from build123d import *

# Parameters (mm, degrees)
BOSS_EXTRUDE1_DEPTH       = 58
SKETCH3_R                 = 2.5
SKETCH3_R_2               = 20
CUT_EXTRUDE1_DEPTH        = 58
SKETCH5_R                 = 3
CUT_EXTRUDE3_DEPTH        = 58
F_4_40_TAPPED_HOLE2_D     = 2.2606
F_4_40_TAPPED_HOLE2_DEPTH = 7.6
F_4_40_TAPPED_HOLE2_TIP   = 0.679152758
SKETCH15_R                = 3
CUT_EXTRUDE4_DEPTH        = 10
FILLET1_R                 = 2
FILLET2_R                 = 2
FILLET3_R                 = 2
FILLET4_R                 = 2


with BuildPart() as part:
    # Sketch2 → Boss-Extrude1 (new body)
    with BuildSketch(Plane.XY):
        Polygon((2, 51.896715462), (36, 51.896715462), (36, -52.603284538), (75.75, -52.603284538), (75.75, -109.603284538), (72.75, -109.603284538), (72.75, -55.603284538), (33, -55.603284538), (33, 48.896715462), (2, 48.896715462), (-29, 48.896715462), (-29, -55.603284538), (-58, -55.603284538), (-58, -109.603284538), (-61, -109.603284538), (-61, -52.603284538), (-32, -52.603284538), (-32, 51.896715462), align=None)
    extrude(amount=BOSS_EXTRUDE1_DEPTH)

    # Sketch3 → Cut-Extrude1 (cut)
    with BuildSketch(Plane(origin=(0, 51.896715462, 0), x_dir=(1, 0, 0), z_dir=(0, 1, 0))):
        with Locations((-21.5, -5.5)):
            Circle(SKETCH3_R)
        with Locations((21.5, -5.5)):
            Circle(SKETCH3_R)
        with Locations((21.5, -52.5)):
            Circle(SKETCH3_R)
        with Locations((-21.5, -52.5)):
            Circle(SKETCH3_R)
        with Locations((2, -29)):
            Circle(SKETCH3_R_2)
    extrude(amount=-CUT_EXTRUDE1_DEPTH, mode=Mode.SUBTRACT)

    # Sketch5 → Cut-Extrude3 (cut)
    with BuildSketch(Plane.ZY.offset(61)):
        with Locations((29, -96.903284538)):
            Circle(SKETCH5_R)
    extrude(amount=-CUT_EXTRUDE3_DEPTH, mode=Mode.SUBTRACT)

    # #4-40 Tapped Hole2
    with Locations(Plane(origin=(75.75, 0, 0), x_dir=(0, 0, -1), z_dir=(1, 0, 0))):
        with Locations((-19.5, -96.902439923), (-24.25, -105.129681259), (-33.75, -105.129681259), (-38.5, -96.902439923), (-33.75, -88.675198587), (-24.25, -88.675198587)):
            Hole(F_4_40_TAPPED_HOLE2_D / 2, depth=F_4_40_TAPPED_HOLE2_DEPTH)
            with Locations((0, 0, -(F_4_40_TAPPED_HOLE2_DEPTH + F_4_40_TAPPED_HOLE2_TIP / 2))):  # 118° drill point
                Cone(0, F_4_40_TAPPED_HOLE2_D / 2, F_4_40_TAPPED_HOLE2_TIP, mode=Mode.SUBTRACT)

    # Sketch15 → Cut-Extrude4 (cut)
    with BuildSketch(Plane(origin=(75.75, 0, 0), x_dir=(0, 0, -1), z_dir=(1, 0, 0))):
        with Locations((-29, -96.902439923)):
            Circle(SKETCH15_R)
    extrude(amount=-CUT_EXTRUDE4_DEPTH, mode=Mode.SUBTRACT)

    # Fillet1
    fillet1_edges = [part.edges().sort_by_distance(p)[0] for p in [
        (36, -0.353284538, 58),
    ]]
    fillet(fillet1_edges, radius=FILLET1_R)

    # Fillet2
    fillet2_edges = [part.edges().sort_by_distance(p)[0] for p in [
        (36, -0.353284538, 0),
    ]]
    fillet(fillet2_edges, radius=FILLET2_R)

    # Fillet3
    fillet3_edges = [part.edges().sort_by_distance(p)[0] for p in [
        (-32, -0.353284538, 0),
    ]]
    fillet(fillet3_edges, radius=FILLET3_R)

    # Fillet4
    fillet4_edges = [part.edges().sort_by_distance(p)[0] for p in [
        (-32, -0.353284538, 58),
    ]]
    fillet(fillet4_edges, radius=FILLET4_R)


solid = part.part
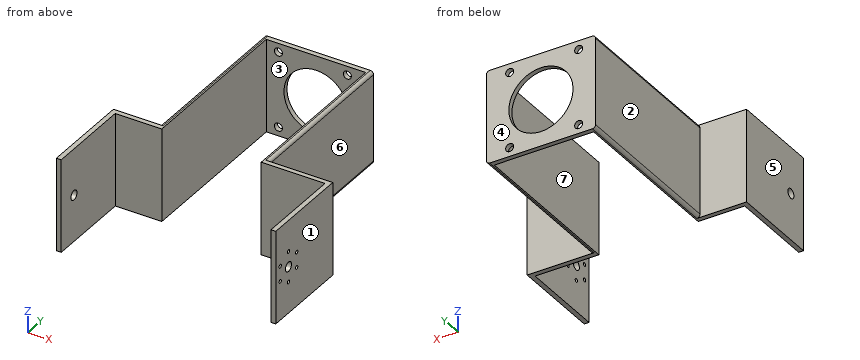
Source: CAD feature listing. Evaluate the final solid. Frame: model axes, mm. Face numbers are marked on the shaded views. A direction names the side the tool comes from. Coordinates: 2 decimals unless noted, no trailing zeros. Write each loop counter-clockwise with the first axis right and the second up, starting at its lowest first coordinate (ties: lowest second). Pieces come first, ordered by that corner, then holes. Notation, with made-up numbers: M 50,65 L 68,65 A21 cw 68,93 Z; hole C 76.5,1.5 d10. An arc over 180 degrees is marked long. Use a Markdown table: item, result.
1) Section D-D, the plane x = 2. Output: boundary loops of the cut face in (y, z), then the cut area to 3 significant figures.
Conclusion:
| item | result |
|---|---|
| outline | M 48.9,0 L 51.9,0 L 51.9,9 L 48.9,9 Z; M 48.9,49 L 51.9,49 L 51.9,58 L 48.9,58 Z |
| area | 54.0 mm^2 |
2) Mould query, pull axis X, two halves, no side actions, for the marked faces 4, 5, 6 and 7. Classes: pulls with the +X half, pulls with the -X half, needs draft (parallel to the pull), parting line crosses it, or undercut.
Conclusion:
| item | result |
|---|---|
| face 4 | needs draft |
| face 5 | pulls with the -X half |
| face 6 | pulls with the +X half |
| face 7 | undercut |
3) Ray query, L1, parallel to X at y = 49.55, z = 5.5; L2, parallel to X at y = 42.5, z = 55.5; L3, parallel to X at y = -67, z = 9. Return the intervals inside material, ascending.
Conclusion:
| item | result |
|---|---|
| L1 | x = -32 to -24, -19 to 19, 24 to 36 |
| L2 | x = -32 to -29, 33 to 36 |
| L3 | x = -61 to -58, 72.75 to 75.75 |
4) Reachability of the marked faces 1, 2 and 3 from +Z, -Z, +X, -X, +Y, -Y: full face, straight path, thin tool, end or side. Return the list, or none.
Conclusion:
| item | result |
|---|---|
| face 1 | +Z, -Z, +X, +Y, -Y |
| face 2 | +Z, -Z, -X, +Y |
| face 3 | +Z, -Z, -Y |
5) Section A-A, the plane y = -62. Output: boundary loops of the cut face in (x, z).
Conclusion:
| item | result |
|---|---|
| outline | M -61,0 L -58,0 L -58,58 L -61,58 Z; M 72.75,0 L 75.75,0 L 75.75,58 L 72.75,58 Z |
6) Section B-B, the plane z = 52.5. Output: boundary loops of the cut face in (x, y), then the cut area to 3 significant figures.
Conclusion:
| item | result |
|---|---|
| outline | M -61,-109.6 L -58,-109.6 L -58,-55.6 L -29,-55.6 L -29,48.9 L -24,48.9 L -24,51.9 L -32,51.9 L -32,-52.6 L -61,-52.6 Z; M -19,48.9 L 19,48.9 L 19,51.9 L -19,51.9 Z; M 24,48.9 L 33,48.9 L 33,-55.6 L 72.75,-55.6 L 72.75,-109.6 L 75.75,-109.6 L 75.75,-52.6 L 36,-52.6 L 36,51.9 L 24,51.9 Z |
| area | 1,330 mm^2 |
7) Section C-C, the plane x = -21.5. Output: boundary loops of the cut face in (y, z).
Conclusion:
| item | result |
|---|---|
| outline | M 48.9,0 L 51.9,0 L 51.9,3 L 48.9,3 Z; M 48.9,8 L 51.9,8 L 51.9,50 L 48.9,50 Z; M 48.9,55 L 51.9,55 L 51.9,58 L 48.9,58 Z |
8) First-contact query: pin 1 Ø3 at (y, z) = (-34.5, 51) entering from +X; pin 2 Ø1.8 at (y, z) = (-96.9, 38.5) entering from +X; pin 3 Ø12.5 at (x, z) = (61.5, 31) entering from +Y. Flat tips, straight axial feed; report the tip coordinate or a pass-through.
Conclusion:
| item | result |
|---|---|
| pin 1 | stops at x = 36 |
| pin 2 | stops at x = -58 |
| pin 3 | stops at y = -52.6 |
